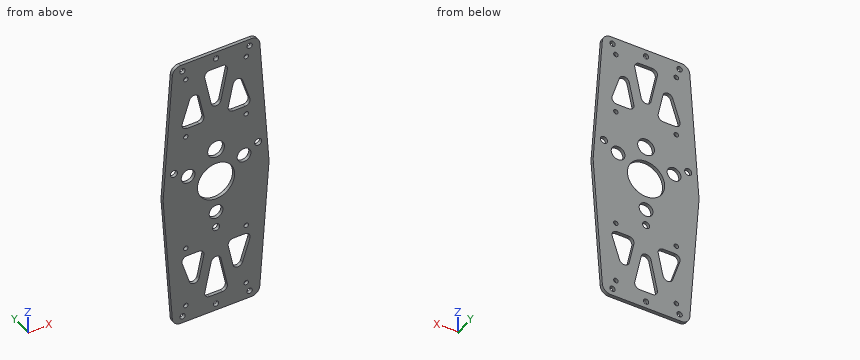
from build123d import *

# Parameters (mm, degrees)
SKETCH_1_W          = 150
SKETCH_1_H          = 180
SKETCH_1_R          = 2.1
EXTRUDE_1_DEPTH     = 2
SKETCH_2_R          = 11.1
SKETCH_2_R_2        = 2.1
SKETCH_2_R_3        = 4.1
SKETCH_2_R_4        = 5
CUT_EXTRUDE_1_DEPTH = 2
SKETCH_3_R          = 1.6
CUT_EXTRUDE_2_DEPTH = 3
SKETCH_4_W          = 150
SKETCH_4_H          = 180
CUT_EXTRUDE_3_DEPTH = 3
FILLET_1_R          = 5
SKETCH_7_R          = 1.35
CUT_EXTRUDE_5_DEPTH = 3
CUT_EXTRUDE_6_DEPTH = 3
FILLET_2_R          = 3


with BuildPart() as part:
    # 草图1 → 凸台-拉伸1 (new body)
    with BuildSketch(Plane(origin=(0, 0, 0), x_dir=(1, 0, 0), z_dir=(0, 1, 0))):
        Rectangle(SKETCH_1_W, SKETCH_1_H)
        with Locations((-70, 85)):
            Circle(SKETCH_1_R, mode=Mode.SUBTRACT)
        with Locations((-50, 85)):
            Circle(SKETCH_1_R, mode=Mode.SUBTRACT)
        with Locations((-50, 65)):
            Circle(SKETCH_1_R, mode=Mode.SUBTRACT)
        with Locations((-70, 65)):
            Circle(SKETCH_1_R, mode=Mode.SUBTRACT)
        with Locations((70, 65)):
            Circle(SKETCH_1_R, mode=Mode.SUBTRACT)
        with Locations((50, 65)):
            Circle(SKETCH_1_R, mode=Mode.SUBTRACT)
        with Locations((50, 85)):
            Circle(SKETCH_1_R, mode=Mode.SUBTRACT)
        with Locations((70, 85)):
            Circle(SKETCH_1_R, mode=Mode.SUBTRACT)
        with Locations((70, -85)):
            Circle(SKETCH_1_R, mode=Mode.SUBTRACT)
        with Locations((50, -85)):
            Circle(SKETCH_1_R, mode=Mode.SUBTRACT)
        with Locations((50, -65)):
            Circle(SKETCH_1_R, mode=Mode.SUBTRACT)
        with Locations((70, -65)):
            Circle(SKETCH_1_R, mode=Mode.SUBTRACT)
        with Locations((-70, -65)):
            Circle(SKETCH_1_R, mode=Mode.SUBTRACT)
        with Locations((-50, -65)):
            Circle(SKETCH_1_R, mode=Mode.SUBTRACT)
        with Locations((-50, -85)):
            Circle(SKETCH_1_R, mode=Mode.SUBTRACT)
        with Locations((-70, -85)):
            Circle(SKETCH_1_R, mode=Mode.SUBTRACT)
    extrude(amount=EXTRUDE_1_DEPTH)

    # 草图2 → 切除-拉伸1 (cut)
    with BuildSketch(Plane(origin=(0, 2, 0), x_dir=(1, 0, 0), z_dir=(0, 1, 0))):
        Circle(SKETCH_2_R)
        with Locations((0, 29)):
            Circle(SKETCH_2_R_2)
        with Locations((25.11473671, -14.5)):
            Circle(SKETCH_2_R_2)
        with Locations((-25.11473671, -14.5)):
            Circle(SKETCH_2_R_2)
        with Locations((0, 19.25)):
            Circle(SKETCH_2_R_3)
        with Locations((16.670989023, -9.625)):
            Circle(SKETCH_2_R_3)
        with Locations((-16.670989023, -9.625)):
            Circle(SKETCH_2_R_3)
        with Locations((0, -20)):
            Circle(SKETCH_2_R_4)
    extrude(amount=-CUT_EXTRUDE_1_DEPTH, mode=Mode.SUBTRACT)

    # 草图3 → 切除-拉伸2 (cut, through all)
    with BuildSketch(Plane(origin=(0, 2, 0), x_dir=(1, 0, 0), z_dir=(0, 1, 0))):
        with Locations((-20, 77)):
            Circle(SKETCH_3_R)
        with Locations((0, 77)):
            Circle(SKETCH_3_R)
        with Locations((20, 77)):
            Circle(SKETCH_3_R)
        with Locations((20, -77)):
            Circle(SKETCH_3_R)
        with Locations((0, -77)):
            Circle(SKETCH_3_R)
        with Locations((-20, -77)):
            Circle(SKETCH_3_R)
    extrude(amount=-CUT_EXTRUDE_2_DEPTH, mode=Mode.SUBTRACT)

    # 草图4 → 切除-拉伸3 (cut, through all)
    with BuildSketch(Plane(origin=(0, 2, 0), x_dir=(1, 0, 0), z_dir=(0, 1, 0))):
        Rectangle(SKETCH_4_W, SKETCH_4_H)
        with BuildLine():
            Line((25.726487009, -81), (-25.726487009, -81))
            Line((-25.726487009, -81), (-31.418007756, -2.271296687))
            ThreePointArc((-31.418007756, -2.271296687), (-31.5, 0), (-31.418007756, 2.271296687))
            Line((-31.418007756, 2.271296687), (-25.726487009, 81))
            Line((-25.726487009, 81), (25.726487009, 81))
            Line((25.726487009, 81), (31.418007756, 2.271296687))
            ThreePointArc((31.418007756, 2.271296687), (31.5, 0), (31.418007756, -2.271296687))
            Line((31.418007756, -2.271296687), (25.726487009, -81))
        make_face(mode=Mode.SUBTRACT)
    extrude(amount=-CUT_EXTRUDE_3_DEPTH, mode=Mode.SUBTRACT)

    # 圆角1
    fillet_1_edges = [part.edges().sort_by_distance(p)[0] for p in [
        (25.726487009, 1, 81),
        (-25.726487009, 1, 81),
        (-25.726487009, 1, -81),
        (25.726487009, 1, -81),
    ]]
    fillet(fillet_1_edges, radius=FILLET_1_R)

    # 草图7 → 切除-拉伸5 (cut, through all)
    with BuildSketch(Plane(origin=(0, 2, 0), x_dir=(1, 0, 0), z_dir=(0, 1, 0))):
        with Locations((-18, 71)):
            Circle(SKETCH_7_R)
        with Locations((18, 71)):
            Circle(SKETCH_7_R)
        with Locations((18, 35)):
            Circle(SKETCH_7_R)
        with Locations((-18, 35)):
            Circle(SKETCH_7_R)
        with Locations((-18, -35)):
            Circle(SKETCH_7_R)
        with Locations((18, -35)):
            Circle(SKETCH_7_R)
        with Locations((18, -71)):
            Circle(SKETCH_7_R)
        with Locations((-18, -71)):
            Circle(SKETCH_7_R)
    extrude(amount=-CUT_EXTRUDE_5_DEPTH, mode=Mode.SUBTRACT)

    # 草图8 → 切除-拉伸6 (cut, through all)
    with BuildSketch(Plane.XZ):
        Polygon((7.5, 71), (-7.5, 71), (0, 36), align=None)
        Polygon((-12.374858275, 67.5), (-21.482001132, 40), (-6.482001132, 40), align=None)
        Polygon((21.482001132, 40), (6.482001132, 40), (12.374858275, 67.5), align=None)
        Polygon((12.374858275, -67.5), (21.482001132, -40), (6.482001132, -40), align=None)
        Polygon((7.5, -71), (-7.5, -71), (0, -36), align=None)
        Polygon((-21.482001132, -40), (-6.482001132, -40), (-12.374858275, -67.5), align=None)
    extrude(amount=-CUT_EXTRUDE_6_DEPTH, mode=Mode.SUBTRACT)

    # 圆角2
    fillet_2_edges = [part.edges().sort_by_distance(p)[0] for p in [
        (-12.374858275, 1, 67.5),
        (-6.482001132, 1, 40),
        (-21.482001132, 1, 40),
        (12.374858275, 1, 67.5),
        (21.482001132, 1, 40),
        (6.482001132, 1, 40),
        (0, 1, -36),
        (7.5, 1, -71),
        (-7.5, 1, -71),
        (12.374858275, 1, -67.5),
        (6.482001132, 1, -40),
        (21.482001132, 1, -40),
        (-12.374858275, 1, -67.5),
        (-21.482001132, 1, -40),
        (-6.482001132, 1, -40),
        (0, 1, 36),
        (-7.5, 1, 71),
        (7.5, 1, 71),
    ]]
    fillet(fillet_2_edges, radius=FILLET_2_R)


solid = part.part
Part model, mm, in its own coordinate system. Coordinates: 2 decimals unless noted, no trailing zeros. Write each loop counter-clockwise with the first axis right and the second up, starting at its lowest first coordinate (ties: lowest second). Pieces come first, ordered by that corner, then holes. Notation, with made-up numbers: M 83.25,1.25 L 126.25,1.25 A19 cw 126.25,13.25 Z; hole C 43.25,31.25 d2. An arc over 180 degrees is marked long. Return JSON: item names as keys, results as strings.
1. Saw through at B-B, the plane x = 24.5. Write the cut outline in (y, z), then the cut area to 3 significant figures.
Determined:
{"outline": "M 0,-79.64 L 2,-79.64 L 2,12.49 L 0,12.49 Z; M 0,16.51 L 2,16.51 L 2,79.64 L 0,79.64 Z", "area": "311 mm²"}
2. Probe L1, parallel to X at y = 0.2, z = 14.5; L2, parallel to X at y = 0.2, z = -52.5; L3, parallel to Z at x = -12, y = 1.7. List the from-to ranges inside material, lowest first.
Determined:
{"L1": "-30.53 to -27.21, -23.01 to 23.01, 27.21 to 30.53", "L2": "-27.79 to -17.34, -9.16 to -3.54, 3.54 to 9.16, 17.34 to 27.79", "L3": "-81 to -58.91, -40 to 40, 58.91 to 81"}
3. Saw through at A-A, the plane z = -19.25. Write the cut outline in (x, y).
Determined:
{"outline": "M -30.19,0 L -4.1,0 L -4.1,2 L -30.19,2 Z; M 4.1,0 L 30.19,0 L 30.19,2 L 4.1,2 Z"}
4. Flat gauge pin, fed straight in: pin 1 Ø1 at (y, z) = (1, 0.5) entering from +X. Where does the tip first touch, or does it go through?
Determined:
{"pin 1": "x = 31.5"}
5. Saw through at C-C, the plane y = 0.5. Count the separate pieces of the cut face and the enclosed holes in it, then the cut area to 3 significant figures.
Determined:
{"separate pieces": "1", "enclosed holes": "28", "area": "7,340 mm²"}
